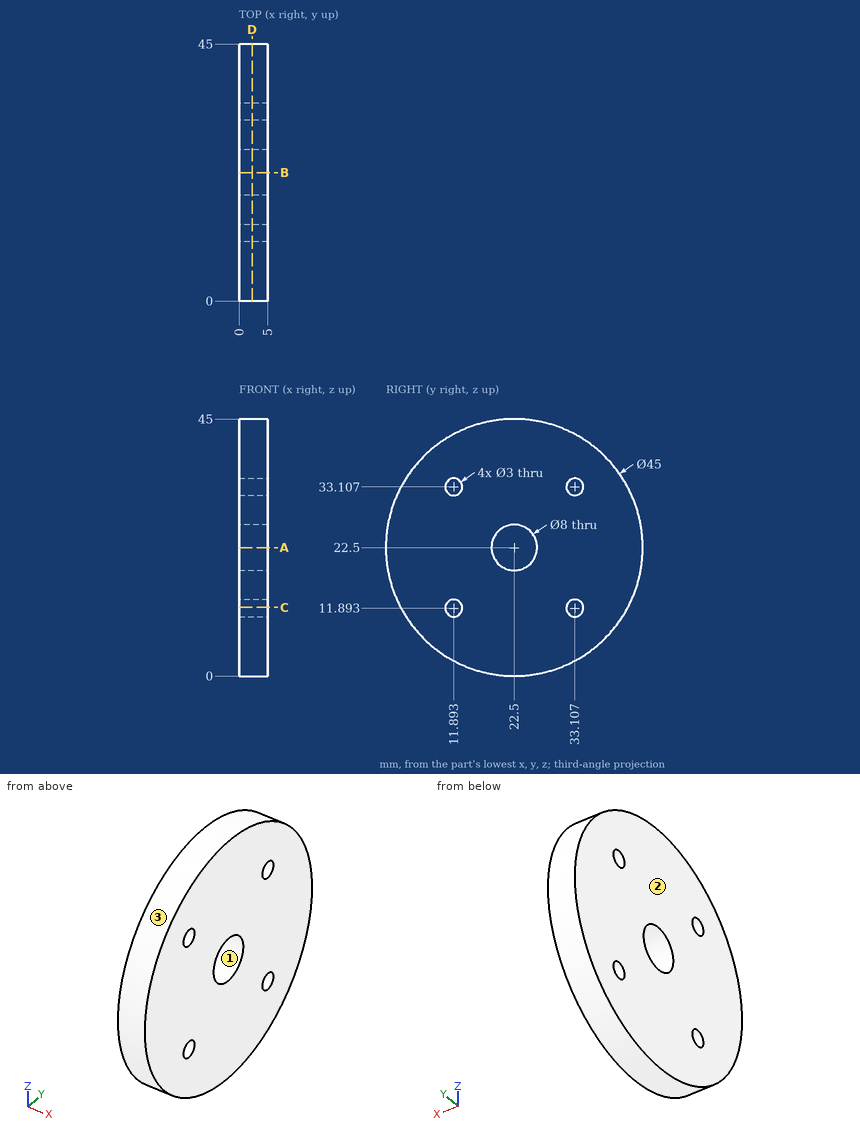
The figure shows three views and two pictorial views of one solid part (mm, origin at its lowest corner). Answer the questions. Give positions to 0.01 mm unless a question says otherwise; leave off trailing zeros. Order: outer loops, then holes, each group sorted by start corner. A loop starts at its lowest first (then second) coordinate and runs counter-clockwise, first axis right, second up. Notation, with made-up numbers: (-33.5, 83.5) -> (25.5, 83.5) arc R25 cw to (25.5, 96.5) -> close; hole circle Ø2 at (88.5, -11). An arc over 180 degrees is marked (long way). Answer as a JSON object with one key per item and string values. Group by question number.
Item 1: Determine the mould class of the marked faces 1, 2 and 3 for opening direction Y: pulls with the +Y half, pulls with the -Y half, needs draft (parallel to the pull), parting line crosses it, or undercut.
Item 2: Flat-ended cylindrical pins translate along their axes: pin 1 (1.5 mm diameter, centred on y = 39, z = 8, fed in from -X); pin 2 (2 mm diameter, centred on x = 2.5, z = 8.5, fed in from -Y) (1 decimal); pin 3 (2 mm diameter, centred on x = 1.5, y = 34, fed in from -Z). Find the tip coordinate at first contact, or state that the pin passes through.
Item 3: Consider L1, parallel to Y at x = 1.6, z = 12.5 (1 decimal); L2, parallel to Z at x = 0.45, y = 34; L3, parallel to Y at x = 2.15, z = 22.5. Determine where each line is inside the solid, lowest interval first. Write a range as from..to.
Item 4: The part is cut by section C-C on z = 12. Write down the section's boundary in (x, y).
Item 5: The part is cut by section A-A on z = 22.5. Write down the section's boundary in (x, y).
Item 6: The part is cut by section D-D on x = 2.25. Write down the section's boundary in (y, z), and give its area (3 significant figures).
Result set:
{
 "1": {"face 1": "undercut", "face 2": "needs draft", "face 3": "parting line crosses it"},
 "2": {"pin 1": "x = 0", "pin 2": "y = 4.1", "pin 3": "z = 2.6"},
 "3": {"L1": "2.3..10.5, 13.3..31.7, 34.5..42.7", "L2": "3.16..10.69, 13.1..31.9, 34.31..41.84", "L3": "0..18.5, 26.5..45"},
 "4": {"outline": "(0, 2.6) -> (5, 2.6) -> (5, 10.4) -> (0, 10.4) -> close; (0, 13.39) -> (5, 13.39) -> (5, 31.61) -> (0, 31.61) -> close; (0, 34.6) -> (5, 34.6) -> (5, 42.4) -> (0, 42.4) -> close"},
 "5": {"outline": "(0, 0) -> (5, 0) -> (5, 18.5) -> (0, 18.5) -> close; (0, 26.5) -> (5, 26.5) -> (5, 45) -> (0, 45) -> close"},
 "6": {"outline": "circle Ø45 at (22.5, 22.5); hole circle Ø3 at (11.89, 11.89); hole circle Ø3 at (11.89, 33.11); hole circle Ø8 at (22.5, 22.5); hole circle Ø3 at (33.11, 11.89); hole circle Ø3 at (33.11, 33.11)", "area": "1,510 mm²"}
}
